```python
from build123d import *

# Parameters (mm, degrees)
F0_W     = 67.056006
F0_H     = 99.669606
F1_DEPTH = 3.55
F2_R     = 5.08
F3_T     = -2.54


with BuildPart() as f1:
    # F0 (on Front) → F1 (new body, symmetric)
    with BuildSketch(Plane.XZ):
        with Locations((-0.489677, 0)):
            Rectangle(F0_W, F0_H)
    extrude(amount=F1_DEPTH, both=True)

    # F2
    f2_edges = [f1.edges().sort_by_distance(p)[0] for p in [
        (-34.01768, 0, -49.834803),
        (-34.01768, 0, 49.834803),
        (33.038326, 0, -49.834803),
        (33.038326, 0, 49.834803),
    ]]
    fillet(f2_edges, radius=F2_R)

    # F3
    f3_openings = [f1.faces().sort_by_distance(p)[0] for p in [
        (-0.489677, -3.55, 0),
    ]]
    offset(amount=F3_T, openings=f3_openings)


solid = f1.part
```
Input: part model. Units: mm. Frame: model coordinates. A direction names the side the tool comes from. Give positions to 0.01 mm unless a question says otherwise; leave off trailing zeros. Loops run counter-clockwise (first coordinate to the right, second up) from the corner with the lowest first, then second, coordinate; pieces in that order, holes last.
1) Line query: L1, parallel to Z at x = -23.5, y = 0.5; L2, parallel to X at y = -2, z = 21.5; L3, parallel to Y at x = 1.5, z = -22. Output: solid intervals per line, ascending.
A:
L1: z = -49.83 to -47.29, 47.29 to 49.83
L2: x = -34.02 to -31.48, 30.5 to 33.04
L3: y = 1.01 to 3.55
2) Section query B-B on x = 26.5. Return the cut outline in (y, z), and give its area (3 significant figures).
A:
outline: (-3.55, -49.83) - (3.55, -49.83) - (3.55, 49.83) - (-3.55, 49.83) - (-3.55, 47.29) - (1.01, 47.29) - (1.01, -47.29) - (-3.55, -47.29) - close
area: 276 mm2
3) Section query A-A on y = -1. Return the cut outline in (x, z).
A:
outline: (-34.02, -44.75) arc R5.08 ccw to (-28.94, -49.83) - (27.96, -49.83) arc R5.08 ccw to (33.04, -44.75) - (33.04, 44.75) arc R5.08 ccw to (27.96, 49.83) - (-28.94, 49.83) arc R5.08 ccw to (-34.02, 44.75) - close; hole (-31.48, -44.75) arc R2.54 ccw to (-28.94, -47.29) - (27.96, -47.29) arc R2.54 ccw to (30.5, -44.75) - (30.5, 44.75) arc R2.54 ccw to (27.96, 47.29) - (-28.94, 47.29) arc R2.54 ccw to (-31.48, 44.75) - close
4) Contact query for a flat-ended pin moving along its axis: pin 1 (2 mm diameter, centred on x = -21, z = -25.5, fed in from -Y). Output: stop coordinate, or through.
A:
pin 1: stops at y = 1.01
5) Mould query, pull axis X, two halves, no side actions, for faces 1 (the cylindrical face through (29.774, -1.302, -46.531)), 2 (the flat face through (-1, 0, 49.835)), 3 (the cylindrical face through (31.59, -0.05, -48.307)). Classes: released by +X, released by -X, zero draft, split by the parting line, or undercut.
A:
face 1: undercut
face 2: zero draft
face 3: released by +X
6) Section query C-C on z = 6. Return the cut outline in (x, y), and give its area (3 significant figures).
A:
outline: (-34.02, -3.55) - (-31.48, -3.55) - (-31.48, 1.01) - (30.5, 1.01) - (30.5, -3.55) - (33.04, -3.55) - (33.04, 3.55) - (-34.02, 3.55) - close
area: 193 mm2
7) Reachability of faces 4 (the flat face through (-1, -1, 47.295)), 5 (the flat face through (-1, 3.55, 1)) from +Z, -Z, +X, -X, +Y, -Y: full face, straight path, thin tool, end or side. Return the list, or none.
A:
face 4: -Y
face 5: +Z, -Z, +X, -X, +Y
